Could you check a few things on this drawing? It's one solid part, dimensions in mm from its lowest x, y, z. A direction names the side the tool comes from. Coordinates: 2 decimals unless noted, no trailing zeros. Write each loop counter-clockwise with the first axis right and the second up, starting at its lowest first coordinate (ties: lowest second). Pieces come first, ordered by that corner, then holes. Notation, with made-up numbers: (-36, 52) - (-10, 52) arc R22 ccw to (-10, 73) - close; hole circle Ø3 at (8, 0.5). An arc over 180 degrees is marked (long way). Use one line per item in the form item = value. Start each with the question number.
(1) If we section it at C-C on z = 11: Please give me the cut outline in (x, y), then the cut area to 3 significant figures.
(2) On a 3-axis mill with a long thin cutter (end or side, diameter ignored), from which of +Z, -Z, +X, -X, +Y, -Y can I reach the whole of each face in a straight line? I mean the marked faces 1 and 2. Say none if no direction works.
(3) If we section it at A-A on x = 11.5: Please give me the cut outline in (y, z) (3 decimals).
(4) If we section it at D-D on x = 3: Please give me the cut outline in (y, z), then the cut area to 3 significant figures.
(5) If I drill on probe 1 along Z at (x, y) = (6.5, 1.25); probe 2 along Y at (x, z) = (14.5, 10.5); probe 3 along X at (y, z) = (8, 13.25), over which ranges is the centre line in solid material (lowest first)? Write a range as from..to.
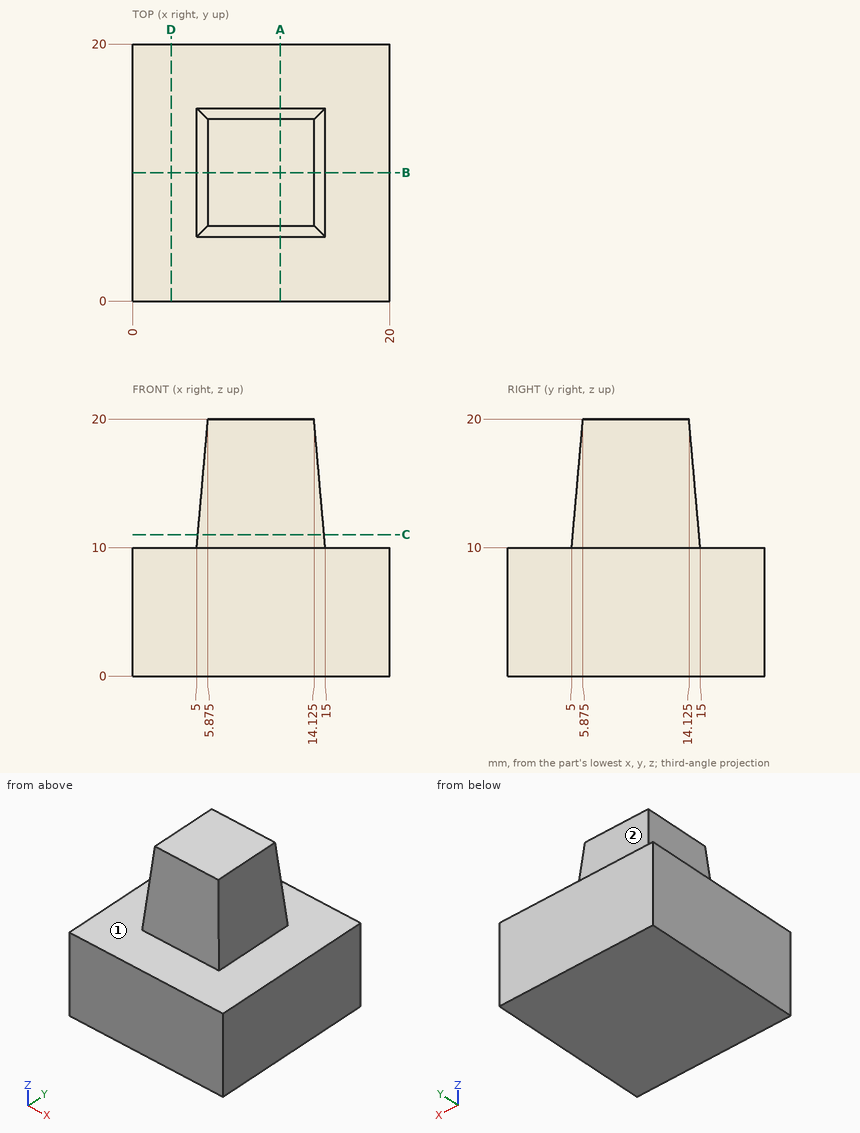
Reported:
q1.outline = (5.09, 5.09) - (14.91, 5.09) - (14.91, 14.91) - (5.09, 14.91) - close
q1.area = 96.5 mm2
q2.face_1 = +Z
q2.face_2 = +Z, +X, -X, +Y
q3.outline = (0, 0) - (20, 0) - (20, 10) - (15, 10) - (14.125, 20) - (5.875, 20) - (5, 10) - (0, 10) - close
q4.outline = (0, 0) - (20, 0) - (20, 10) - (0, 10) - close
q4.area = 200 mm2
q5.probe_1 = 0..10
q5.probe_2 = 5.04..14.96
q5.probe_3 = 5.28..14.72
